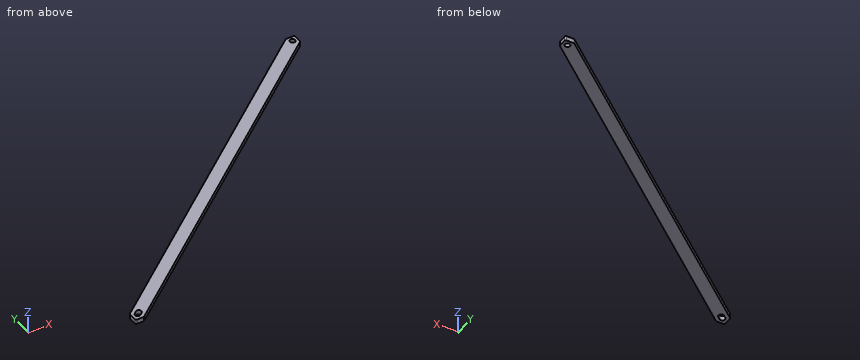
```python
from build123d import *

# Parameters (mm, degrees)
SKETCH_R  = 4.5
PAD_DEPTH = 8


with BuildPart() as part:
    # Sketch → Pad (new body)
    with BuildSketch(Plane.XY):
        with BuildLine():
            Line((-34.918649, 618.551784), (-573.934055, 180.286922))
            ThreePointArc((-573.934055, 180.286922), (-574.47835, 179.594363), (-574.672324, 178.735138))
            Line((-574.672324, 178.735138), (-574.672324, 164.892597))
            ThreePointArc((-574.672324, 164.892597), (-574.086537, 163.478383), (-572.672324, 162.892597))
            Line((-561.164831, 162.892597), (-572.672324, 162.892597))
            ThreePointArc((-561.164831, 162.892597), (-560.495341, 163.007979), (-559.903099, 163.340812))
            Line((-559.903099, 163.340812), (-19.738269, 602.540254))
            ThreePointArc((-19.738269, 602.540254), (-19.193974, 603.232813), (-19, 604.092038))
            Line((-19, 604.092038), (-19, 617))
            ThreePointArc((-19, 617), (-19.585786, 618.414214), (-21, 619))
            Line((-33.656918, 619), (-21, 619))
            ThreePointArc((-33.656918, 619), (-34.326407, 618.884618), (-34.918649, 618.551784))
        make_face()
        with Locations((-28, 610)):
            Circle(SKETCH_R, mode=Mode.SUBTRACT)
        with BuildLine():
            Line((-563.511219, 180.384111), (-568.166572, 176.598918))
            ThreePointArc((-568.166572, 176.598918), (-568.819191, 170.268508), (-562.488781, 169.615889))
            Line((-557.833428, 173.401082), (-562.488781, 169.615889))
            ThreePointArc((-557.833428, 173.401082), (-557.180809, 179.731492), (-563.511219, 180.384111))
        make_face(mode=Mode.SUBTRACT)
    extrude(amount=PAD_DEPTH)


solid = part.part
```
Input: part model. Units: mm. Frame: model coordinates. Coordinates: 2 decimals unless noted, no trailing zeros. Write each loop counter-clockwise with the first axis right and the second up, starting at its lowest first coordinate (ties: lowest second). Pieces come first, ordered by that corner, then holes. Notation, with made-up numbers: (-38, -39.75) -> (8, -39.75) arc R21 ccw to (8, -17.75) -> close; hole circle Ø7 at (19.25, 35). An arc over 180 degrees is marked (long way). Write each question's results on one line, items separated by ' | '.
Item 1: Section query A-A on z = 2.75. Return loops of the section in (x, y), plus the area to 3 significant figures.
Conclusion:
outline: (-574.67, 164.89) arc R2 ccw to (-572.67, 162.89) -> (-561.16, 162.89) arc R2 ccw to (-559.9, 163.34) -> (-19.74, 602.54) arc R2 ccw to (-19, 604.09) -> (-19, 617) arc R2 ccw to (-21, 619) -> (-33.66, 619) arc R2 ccw to (-34.92, 618.55) -> (-573.93, 180.29) arc R2 ccw to (-574.67, 178.74) -> close; hole (-568.17, 176.6) arc R4.5 ccw to (-562.49, 169.62) -> (-557.83, 173.4) arc R4.5 ccw to (-563.51, 180.38) -> close; hole circle Ø9 at (-28, 610) | area: 15,400 mm^2
Item 2: Material intervals for probe 1 along X at (y, z) = (610, 4); probe 2 along Y at (x, z) = (-63, 1.25); probe 3 along Y at (x, z) = (-477.5, 2.5), sorted ascending.
Conclusion:
probe 1: x = -45.44 to -32.5, -23.5 to -19 | probe 2: y = 567.36 to 595.72 | probe 3: y = 230.34 to 258.7
Item 3: Pin query (flat end, axial travel): pin 1 Ø4 at (y, z) = (255, 5) entering from -X; pin 2 Ø5.5 at (x, y) = (-28, 610) entering from -Z. Return the tip coordinate at first contact, or that it passes through.
Conclusion:
pin 1: stops at x = -484.51 | pin 2: passes through
Item 4: Section query B-B on x = -98. Return loops of the section in (y, z).
Conclusion:
outline: (538.91, 0) -> (567.26, 0) -> (567.26, 8) -> (538.91, 8) -> close
Item 5: Section query C-C on y = 438.5. Return loops of the section in (x, z).
Conclusion:
outline: (-256.36, 0) -> (-221.49, 0) -> (-221.49, 8) -> (-256.36, 8) -> close
